Job drawing, mm, ordinate dimensions from the low corner. One solid piece. Coordinates: 2 decimals unless noted, no trailing zeros. Write each loop counter-clockwise with the first axis right and the second up, starting at its lowest first coordinate (ties: lowest second). Pieces come first, ordered by that corner, then holes. Notation, with made-up numbers: (-35, -17) - (9, -17) arc R20 ccw to (9, 15) - close; hole circle Ø6 at (1, 21.25). An arc over 180 degrees is marked (long way). Put each result on its own line as item: value. Start each with the question number.
1. Drill centre lines: L1, parallel to Y at x = 8.5, z = 34.5 (1 decimal); L2, parallel to Y at x = 1, z = 33 (1 decimal); L3, parallel to Y at x = 4.75, z = 11.5 (1 decimal). Where is each one in solid material? Low to high. Write a range as from..to.
2. Saw through at D-D, the plane z = 21.5. Write the cut outline in (x, y).
3. Pull direction Y, two halves, no side cores. Call the marked faces 1, 2 and 3: released by +Y, released by -Y, zero draft, split by the parting line, or undercut.
4. Drop a flat-ended pin along its axis: P1, Ø12, axis at y = 16.5, z = 8, coming from the -X side. Give the stop position or say it passes through.
5. Saw through at C-C, the plane x = 7.25. Write the cut outline in (y, z) (1 decimal).
6. Saw through at A-A, the plane x = 12.75. Write the cut outline in (y, z) (1 decimal), plus the area to 3 significant figures.
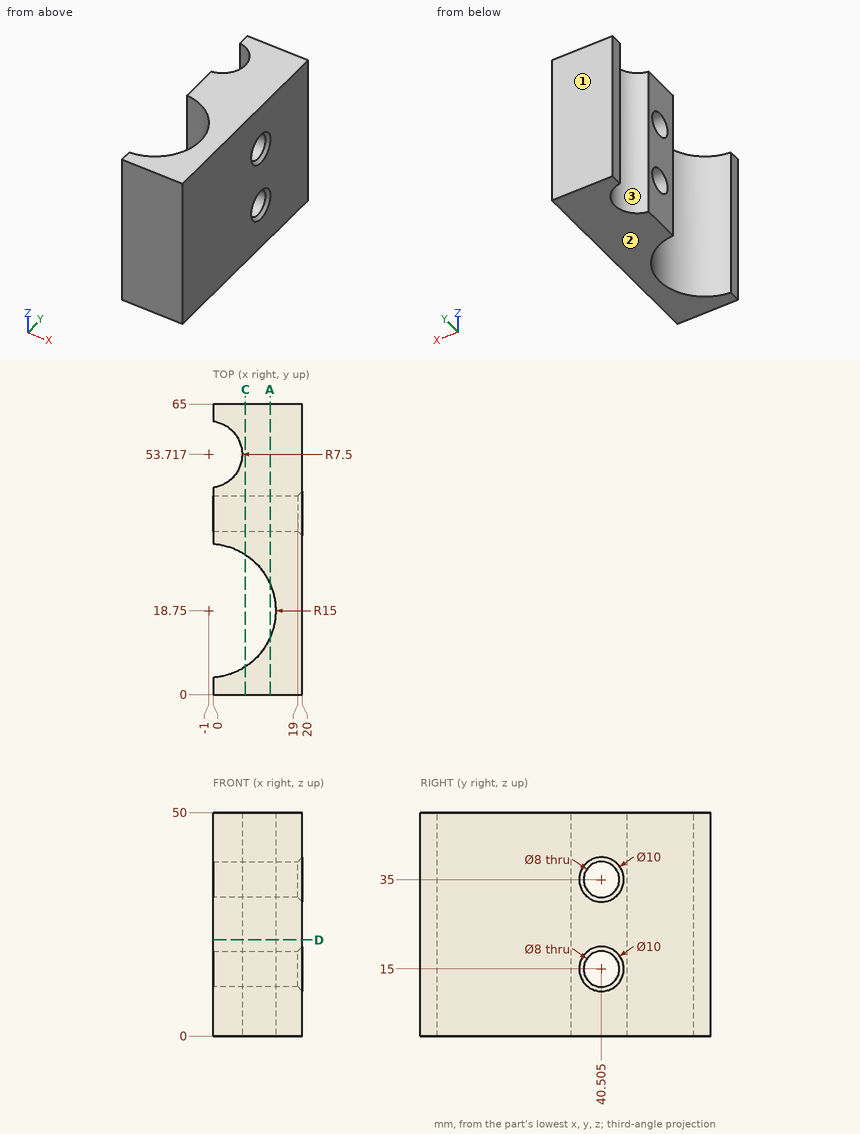
Final values:
1. L1: y = 0..7.1, 30.4..36.5, 44.5..65
1. L2: y = 0..3.9, 33.6..37, 44..46.5, 60.9..65
1. L3: y = 0..4.9, 32.6..38.6, 42.4..48.9, 58.5..65
2. outline: (0, 0) - (20, 0) - (20, 65) - (0, 65) - (0, 61.15) arc R7.5 cw to (0, 46.28) - (0, 33.72) arc R15 cw to (0, 3.78) - close
3. face 1: released by +Y
3. face 2: zero draft
3. face 3: undercut
4. P1: stops at x = 11.53
5. outline: (0, 0) - (6.2, 0) - (6.2, 50) - (0, 50) - close; (31.3, 0) - (65, 0) - (65, 50) - (31.3, 50) - close; hole circle Ø8 at (40.5, 15); hole circle Ø8 at (40.5, 35)
6. outline: (0, 0) - (12.8, 0) - (12.8, 50) - (0, 50) - close; (24.7, 0) - (65, 0) - (65, 50) - (24.7, 50) - close; hole circle Ø8 at (40.5, 15); hole circle Ø8 at (40.5, 35)
6. area: 2,550 mm²
